```python
from build123d import *

# Parameters (mm, degrees)
F1_DEPTH = 180
F3_DEPTH = 10
F5_DEPTH = 25


with BuildPart() as f1:
    # F0 (on Front) → F1 (new body)
    with BuildSketch(Plane.XZ):
        Polygon((56, 0), (0, 0), (0, -5), (-12, -5), (-12, -8), (0, -15.2), (0, -17), (0, -25), (56, -25), align=None)
    extrude(amount=F1_DEPTH)

    # F2 (on face) → F3 (cut)
    with BuildSketch(Plane.XY):
        with BuildLine():
            Line((13.500019, -164.5), (42.466399, -164.499925))
            ThreePointArc((42.466399, -164.499925), (50, -157), (42.466399, -149.500075))
            Line((42.466399, -149.500075), (14.039766, -149.519448))
            ThreePointArc((14.039766, -149.519448), (6.004863, -156.729951), (13.500019, -164.5))
        make_face()
        with BuildLine():
            Line((13.500019, -30.5), (42.466399, -30.499925))
            ThreePointArc((42.466399, -30.499925), (50, -23), (42.466399, -15.500075))
            Line((42.466399, -15.500075), (13.500019, -15.5))
            ThreePointArc((13.500019, -15.5), (6, -23), (13.500019, -30.5))
        make_face()
    extrude(amount=-F3_DEPTH, mode=Mode.SUBTRACT)

    # F4 (on face) → F5 (cut)
    with BuildSketch(Plane.XY):
        with BuildLine():
            Line((42.5, -18), (13.5, -18))
            ThreePointArc((13.5, -18), (8.5, -23), (13.5, -28))
            Line((13.5, -28), (42.5, -28))
            ThreePointArc((42.5, -28), (47.5, -23), (42.5, -18))
        make_face()
        with BuildLine():
            Line((42.5, -152), (13.5, -152))
            ThreePointArc((13.5, -152), (8.5, -157), (13.5, -162))
            Line((13.5, -162), (42.5, -162))
            ThreePointArc((42.5, -162), (47.5, -157), (42.5, -152))
        make_face()
    extrude(amount=-F5_DEPTH, mode=Mode.SUBTRACT)


solid = f1.part
```
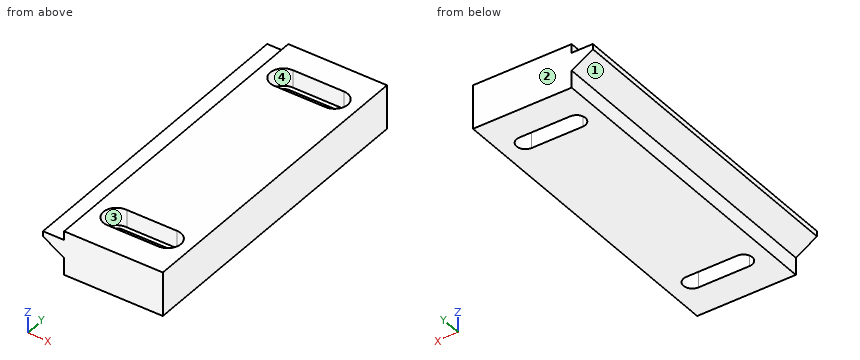
For this review, take the finished solid that the model builds, in its own axes (mm). Face numbers are marked on the shaded views. Round coordinates to 2 decimals unless told otherwise and drop trailing zeros. Write each loop counter-clockwise with the first axis right and the second up, starting at its lowest first coordinate (ties: lowest second). Pieces come first, ordered by that corner, then holes.
1) Take a section at D-D on y = -44.5. Give the boundary of the cut face in (x, z).
Answer below:
outline: (-12, -8) - (0, -15.2) - (0, -25) - (56, -25) - (56, 0) - (0, 0) - (0, -5) - (-12, -5) - close
2) Take a section at A-A on z = -12.5. Give the boundary of the cut face in (x, y).
Answer below:
outline: (-4.5, -180) - (56, -180) - (56, 0) - (-4.5, 0) - close; hole (13.5, -162) - (42.5, -162) arc R5 ccw to (42.5, -152) - (13.5, -152) arc R5 ccw to start; hole (13.5, -28) - (42.5, -28) arc R5 ccw to (42.5, -18) - (13.5, -18) arc R5 ccw to start
3) Mouldability with a two-part tool opening along Y and no side actions: class the marked faces 1, 2, 3 and 4 as +Y half, -Y half, draft (parallel to the pull), parting line (faces both ways), or undercut.
Answer below:
face 1: draft
face 2: +Y half
face 3: undercut
face 4: undercut
4) Take a section at C-C on x = 24.5. Give the boundary of the cut face in (y, z).
Answer below:
outline: (-180, -25) - (-162, -25) - (-162, -10) - (-164.5, -10) - (-164.5, 0) - (-180, 0) - close; (-152, -25) - (-28, -25) - (-28, -10) - (-30.5, -10) - (-30.5, 0) - (-149.51, 0) - (-149.51, -10) - (-152, -10) - close; (-18, -25) - (0, -25) - (0, 0) - (-15.5, 0) - (-15.5, -10) - (-18, -10) - close
5) Insertion check: pin 1 Ø12 at (x, y) = (25, -154) entering from +Z; pin 2 Ø6 at (y, z) = (-70.5, -16.5) entering from -X; pin 3 Ø2 at (y, z) = (-54.5, -16) entering from -X; pin 4 Ø8 at (y, z) = (-121.5, -18) entering from -X. Each pin has a flat end and moves straight along its axis. Give the tip position at first contact, or say it passes through.
Answer below:
pin 1: stops at z = 0
pin 2: stops at x = -2.83
pin 3: stops at x = -0.33
pin 4: stops at x = -2
6) Take a section at B-B on y = -157. Give the boundary of the cut face in (x, z), then the cut area to 3 significant figures.
Answer below:
outline: (-12, -8) - (0, -15.2) - (0, -25) - (8.5, -25) - (8.5, -10) - (6, -10) - (6, 0) - (0, 0) - (0, -5) - (-12, -5) - close; (47.5, -25) - (56, -25) - (56, 0) - (50, 0) - (50, -10) - (47.5, -10) - close
area: 454 mm2
7) For line 1 along Y through (x, z) = (30.5, -9); line 2 along Y through (x, z) = (37, -16.75); line 3 along X through (y, z) = (-111, -21.5), list the stretches that pass through material, from the lowest coordinate up.
Answer below:
line 1: y = -180 to -164.5, -149.51 to -30.5, -15.5 to 0
line 2: y = -180 to -162, -152 to -28, -18 to 0
line 3: x = 0 to 56
